Autodesk Fusion 360 part; units mm, degrees
sketch "Sketch8" plane through (0, 0, 0) normal (0, 0, 1) x (1, 0, 0)
  line L0 (0, 0) -> (20, 0)
  line L1 (20, 0) -> (20, 96)
  line L2 (20, 96) -> (0, 96)
  line L3 (0, 96) -> (0, 0)
  line L4 (0, 48) -> (-20, 48) construction
  line L5 (-20, 48) -> (-20, 58) construction
  line L6 (-20, 58) -> (0, 58)
  line L7 (0, 58) -> (0, 38)
  line L8 (0, 38) -> (-20, 38)
  line L9 (-20, 38) -> (-20, 58)
  line L10 (-20, 58) -> (0, 38) construction
  circle A0 centre (-10, 48) radius 2.5
  line L11 (0, 96) -> (20, 76) construction
  line L12 (0, 96) -> (28.2843, 96) construction
  circle A1 centre (10, 86) radius 2.5
  circle A2 centre (10, 10) radius 2.5
  dimension "d44" = 20
  dimension "d45" = 96
  dimension "d46" = 20
  dimension "d47" = 10
  dimension "d48" = 20
  dimension "d49" = 20
  dimension "d50" = 5
  dimension "d51" = 45
  dimension "d52" = 5
extrude "Extrude10" add sketch "Sketch8" along normal blind 6
sketch "Sketch9" plane through (0, 0, 6) normal (0, 0, 1) x (-1, 0, 0)
  circle A0 centre (10, -48) radius 2.5
  circle A1 centre (-10, -10) radius 2.5
  circle A2 centre (-10, -86) radius 2.5
  line L0 (0, -38) -> (0, 0)
  line L1 (0, 0) -> (-20, 0)
  line L2 (-20, 0) -> (-20, -96)
  line L3 (-20, -96) -> (0, -96)
  line L4 (0, -96) -> (0, -58)
  line L5 (0, -58) -> (20, -58)
  line L6 (20, -58) -> (20, -38)
  line L7 (20, -38) -> (0, -38)
  line L8 (-20, -48) -> (20, -48) construction
  line L9 (-20, -48) -> (-20, -52) construction
  line L10 (-20, -52) -> (-6, -52)
  line L11 (-6, -52) -> (-6, -72.5)
  line L12 (-6, -72.5) -> (-20, -72.5)
  line L13 (-20, -72.5) -> (-20, -52)
  line L14 (-20, -44) -> (-6, -44)
  line L15 (-6, -44) -> (-6, -23.5)
  line L16 (-6, -23.5) -> (-20, -23.5)
  dimension "d55" = 4
  dimension "d57" = 14
  dimension "d58" = 20.5
extrude "Extrude11" add sketch "Sketch9" along normal blind 116.5 contours L2 L14 L15 L16 | L2 L10 L11 L12 L13
sketch "Sketch10" plane through (0, 0, 122.5) normal (0, 0, 1) x (-1, 0, 0)
  line L0 (-6, -23.5) -> (-20, -23.5)
  line L1 (-20, -23.5) -> (-20, -44)
  line L2 (-20, -44) -> (-6, -44)
  line L3 (-6, -44) -> (-6, -23.5)
  line L4 (-20, -72.5) -> (-6, -72.5)
  line L5 (-6, -72.5) -> (-6, -52)
  line L6 (-6, -52) -> (-20, -52)
  line L7 (-20, -52) -> (-20, -72.5)
  line L8 (-6, -72.5) -> (-20, -72.5)
  line L9 (-20, -72.5) -> (-20, -23.5)
  line L10 (-20, -23.5) -> (-6, -23.5)
  line L11 (-6, -23.5) -> (-6, -72.5)
extrude "Extrude12" add sketch "Sketch10" against normal blind 3
sketch "Sketch11" plane through (20, 0, 0) normal (1, 0, 0) x (0, 1, 0)
  line L0 (52, 119.5) -> (52, 6)
  line L1 (52, 6) -> (44, 6)
  line L2 (44, 6) -> (44, 119.5)
  line L3 (72.5, 122.5) -> (23.5, 122.5)
  line L4 (72.5, 6) -> (72.5, 122.5)
  line L5 (44, 119.5) -> (52, 119.5)
  line L6 (23.5, 122.5) -> (23.5, 6)
  line L7 (23.5, 6) -> (0, 6)
  line L8 (0, 6) -> (0, 0)
  line L9 (0, 0) -> (96, 0)
  line L10 (96, 0) -> (96, 6)
  line L11 (96, 6) -> (72.5, 6)
  line L12 (23.5, 6) -> (44, 6) construction
  line L13 (48, 119.5) -> (48, 6) construction
  line L14 (26.5, 119.5) -> (41, 119.5)
  line L15 (41, 119.5) -> (41, 9)
  line L16 (41, 9) -> (26.5, 9)
  line L17 (26.5, 9) -> (26.5, 119.5)
  line L18 (55, 119.5) -> (55, 9)
  line L19 (69.5, 119.5) -> (55, 119.5)
  line L20 (69.5, 9) -> (69.5, 119.5)
  line L21 (55, 9) -> (69.5, 9)
  dimension "d64" = 3
  dimension "d65" = 3
  dimension "d67" = 3
  dimension "d68" = 3
sketch "Sketch14" plane through (6, 0, 0) normal (-1, 0, 0) x (0, -1, 0)
  line L0 (-72.5, 122.5) -> (-72.5, 6)
  line L1 (-72.5, 6) -> (-52, 6)
  line L2 (-52, 6) -> (-52, 119.5)
  line L3 (-52, 119.5) -> (-44, 119.5)
  line L4 (-44, 119.5) -> (-44, 6)
  line L5 (-44, 6) -> (-23.5, 6)
  line L6 (-23.5, 6) -> (-23.5, 122.5)
  line L7 (-23.5, 122.5) -> (-72.5, 122.5)
  line L8 (-69.5, 9) -> (-69.5, 119.5)
  line L9 (-55, 9) -> (-69.5, 9)
  line L10 (-55, 119.5) -> (-55, 9)
  line L11 (-69.5, 119.5) -> (-55, 119.5)
  line L12 (-26.5, 119.5) -> (-41, 119.5)
  line L13 (-41, 119.5) -> (-41, 9)
  line L14 (-26.5, 9) -> (-26.5, 119.5)
  line L15 (-41, 9) -> (-26.5, 9)
extrude "Extrude13" cut sketch "Sketch14" against normal blind 11 contours L8 L9 L10 L11 | L12 L13 L14 L15
extrude "Extrude14" add 1 faces at (15.3333, 46.6667, 119.5) along direction (0, 0, -1) up to surface (113.5 mm away)
sketch "Sketch15" plane through (17, 0, 0) normal (-1, 0, 0) x (0, -1, 0)
  line L0 (-69.5, 119.5) -> (-69.5, 9)
  line L1 (-69.5, 9) -> (-55, 9)
  line L2 (-55, 9) -> (-55, 119.5)
  line L3 (-55, 119.5) -> (-69.5, 119.5)
  line L4 (-56, 118.5) -> (-68.5, 118.5)
  line L5 (-68.5, 118.5) -> (-68.5, 10)
  line L6 (-68.5, 10) -> (-56, 10)
  line L7 (-56, 10) -> (-56, 118.5)
extrude "Extrude15" add sketch "Sketch15" along normal blind 8
sketch "Sketch16" plane through (17, 0, 0) normal (-1, 0, 0) x (0, -1, 0)
  line L0 (-41, 9) -> (-26.5, 9)
  line L1 (-26.5, 9) -> (-26.5, 119.5)
  line L2 (-26.5, 119.5) -> (-41, 119.5)
  line L3 (-41, 119.5) -> (-41, 9)
  line L4 (-27.5, 118.5) -> (-40, 118.5)
  line L5 (-40, 118.5) -> (-40, 10)
  line L6 (-40, 10) -> (-27.5, 10)
  line L7 (-27.5, 10) -> (-27.5, 118.5)
extrude "Extrude16" add sketch "Sketch16" along normal blind 8
sketch "Sketch17" plane through (6, 0, 0) normal (-1, 0, 0) x (0, -1, 0)
  line L0 (-55, 9) -> (-69.5, 9)
  line L1 (-69.5, 9) -> (-69.5, 119.5)
  line L2 (-69.5, 119.5) -> (-55, 119.5)
  line L3 (-55, 119.5) -> (-55, 9)
  line L4 (-26.5, 119.5) -> (-26.5, 9)
  line L5 (-26.5, 9) -> (-41, 9)
  line L6 (-41, 9) -> (-41, 119.5)
  line L7 (-41, 119.5) -> (-26.5, 119.5)
  line L8 (-72.5, 6) -> (-23.5, 6)
  line L9 (-23.5, 6) -> (-23.5, 122.5)
  line L10 (-23.5, 122.5) -> (-72.5, 122.5)
  line L11 (-72.5, 122.5) -> (-72.5, 6)
  line L12 (-69.5, 9) -> (-72.5, 9)
  line L13 (-26.5, 9) -> (-23.5, 9)
  line L14 (-26.5, 119.5) -> (-23.5, 119.5)
  line L15 (-69.5, 119.5) -> (-72.5, 119.5)
extrude "Extrude17" cut sketch "Sketch17" against normal blind 2 contours L1 L11 L12 L15 | L4 L9 L13 L14
equation "thickness = 6 mm"
equation "bar_width = 14 mm"
equation "bar_length = 110 mm"
equation "bar_under_depth = 8 mm"
equation "bar_thickness = 3 mm"
equation "bar_shelf_width = 1 mm"
equation "space_between_bars = 8 mm"
equation "frame_width = 96 mm"
equation "extrusion_width = 20 mm"
equation "mounting_hole_size = 5 mm"
equation "d44 = extrusion_width"
equation "d45 = frame_width"
equation "d46 = extrusion_width"
equation "d47 = extrusion_width / 2"
equation "d48 = extrusion_width"
equation "d49 = extrusion_width"
equation "d50 = mounting_hole_size"
equation "d52 = mounting_hole_size"
equation "d53 = thickness"
equation "d55 = space_between_bars / 2"
equation "small_thickness = 3 mm"
equation "d57 = bar_thickness + bar_under_depth + small_thickness"
equation "d58 = bar_width + small_thickness * 2 + tolerance * 2"
equation "tolerance = 0.25 mm"
equation "d60 = bar_length + small_thickness * 2 + tolerance * 2"
equation "d64 = small_thickness"
equation "d65 = small_thickness"
equation "d67 = small_thickness"
equation "d68 = small_thickness"
equation "d74 = bar_under_depth"
equation "d77 = bar_under_depth"
equation "wire_cutout_depth = 2 mm"
Model file for the job. Use its own axes, mm. A direction names the side the tool comes from. Give positions to 0.01 mm unless a question says otherwise; leave off trailing zeros. Write each loop counter-clockwise with the first axis right and the second up, starting at its lowest first coordinate (ties: lowest second). Pieces come first, ordered by that corner, then holes. Notation, with made-up numbers: (-19.75, -5.5) - (9.25, -5.5) arc R15 ccw to (9.25, 21.5) - close; hole circle Ø8 at (1, 34.25). An arc over 180 degrees is marked (long way). One line per question, with ' | ' between items. Start each with the question number.
(1) Slice it at B-B on x = -10. Write the cut outline in (y, z), plus the area to 3 significant figures.
(2) Pin check, flat tips, straight feed: P1, Ø5, axis at y = 69, z = 3.5, coming from the -X side; P2, Ø12, axis at x = 8, z = 62, coming from the -Y side; P3, Ø2.5, axis at y = 24.5, z = 72.5, coming from the -X side. Stop position of each tip, or through.
(3) Slice it at C-C on z = 112. Write the cut outline in (x, y), plus the area to 3 significant figures.
(4) 3-axis set-ups, long thin cutter, end or side, ignore diameter. For faces 1 (the face through (13, 27.5, 63)), 2 (the face through (-10, 38, 3)), 3 (the face through (13, 23.5, 63)): which of +Z, -Z, +X, -X, +Y, -Y reach the whole face in a straight line?
(5) Two-plate mould, pull along X, no slides. Class faces 4 (the face through (9, 40.2, 64.5)), 5 (the face through (9.46, 12.44, 2.96)), 6 (the face through (13, 34, 10)): +X half, -X half, draft (parallel to the pull), parting line (faces both ways), or undercut.
(6) Slice it at D-D on y = 65. Write the cut outline in (x, z).
(7) Wall check: line 1 along Y through (x, z) = (10, 3.4); line 2 along Y through (x, z) = (-10, 1); line 3 along X through (y, z) = (33, 100). Give the ranges that are in metal, low to high. Write a range as from..to.
(8) Slice it at A-A on y = 86. Write the cut outline in (x, z).
Results below:
1) outline: (38, 0) - (45.5, 0) - (45.5, 6) - (38, 6) - close; (50.5, 0) - (58, 0) - (58, 6) - (50.5, 6) - close | area: 90.0 mm^2
2) P1: x = 0 | P2: y = 23.5 | P3: x = 8
3) outline: (6, 41) - (9, 41) - (9, 40) - (17, 40) - (17, 27.5) - (9, 27.5) - (9, 26.5) - (8, 26.5) - (8, 23.5) - (20, 23.5) - (20, 72.5) - (8, 72.5) - (8, 69.5) - (9, 69.5) - (9, 68.5) - (17, 68.5) - (17, 56) - (9, 56) - (9, 55) - (6, 55) - close | area: 387 mm^2
4) face 1: -X | face 2: +Z, -Z, -X, -Y | face 3: +Z, +X, -X, -Y
5) face 4: -X half | face 5: undercut | face 6: draft
6) outline: (0, 0) - (20, 0) - (20, 122.5) - (6, 122.5) - (6, 119.5) - (9, 119.5) - (9, 118.5) - (17, 118.5) - (17, 10) - (9, 10) - (9, 9) - (6, 9) - (6, 6) - (0, 6) - close
7) line 1: 0..7.5, 12.5..83.5, 88.5..96 | line 2: 38..45.5, 50.5..58 | line 3: 17..20
8) outline: (0, 0) - (7.5, 0) - (7.5, 6) - (0, 6) - close; (12.5, 0) - (20, 0) - (20, 6) - (12.5, 6) - close
